```python
from build123d import *

# Parameters (mm, degrees)
SKETCH1_R           = 2
BOSS_EXTRUDE1_DEPTH = 2
SKETCH6_R           = 1.4
CUT_EXTRUDE1_DEPTH  = 10


with BuildPart() as part:
    # Sketch1 → Boss-Extrude1 (new body)
    with BuildSketch(Plane(origin=(0, 0, 0), x_dir=(1, 0, 0), z_dir=(0, 1, 0))):
        with BuildLine():
            ThreePointArc((9.383115236, 31.116027196), (-30.08527478, 12.293341344), (-15.092629238, -28.783025253))
            ThreePointArc((-15.092629238, -28.783025253), (-13.079214236, -32.008527478), (-9.383115236, -31.116027196))
            ThreePointArc((-9.383115236, -31.116027196), (30.08527478, -12.293341344), (15.092629238, 28.783025253))
            ThreePointArc((15.092629238, 28.783025253), (13.079214236, 32.008527478), (9.383115236, 31.116027196))
        make_face()
        with Locations((11.849880102, 29)):
            Circle(SKETCH1_R, mode=Mode.SUBTRACT)
        with Locations((-11.849880102, -29)):
            Circle(SKETCH1_R, mode=Mode.SUBTRACT)
    extrude(amount=BOSS_EXTRUDE1_DEPTH)

    # Sketch6 → Cut-Extrude1 (cut)
    with BuildSketch(Plane.XZ):
        with Locations((-21.83, -13.926611625)):
            Circle(SKETCH6_R)
        with Locations((22.12, 14.29)):
            Circle(SKETCH6_R)
    extrude(amount=-CUT_EXTRUDE1_DEPTH, mode=Mode.SUBTRACT)


solid = part.part
```
CAD build for the part. Positions are in the model's coordinates, mm. Coordinates: 2 decimals unless noted, no trailing zeros. Loops run counter-clockwise (first coordinate to the right, second up) from the corner with the lowest first, then second, coordinate; pieces in that order, holes last. Notation, with made-up numbers: (14.25, 77.25) - (26.25, 77.25) arc R22 ccw to (26.25, 99.25) - close; hole circle Ø7 at (-13, 66). An arc over 180 degrees is marked (long way). Return JSON: item names as keys, results as strings.
1. Band-saw the part on B-B (x = 12). Give the cut face in (y, z), and give its area (3 significant figures).
Result:
{"outline": "(0, -32.25) - (2, -32.25) - (2, -30.99) - (0, -30.99) - close; (0, -27.01) - (2, -27.01) - (2, 30.2) - (0, 30.2) - close", "area": "117 mm2"}
2. Band-saw the part on A-A (z = 14.29). Give the cut face in (x, y), and give its area (3 significant figures).
Result:
{"outline": "(-29.19, 0) - (20.72, 0) - (20.72, 2) - (-29.19, 2) - close; (23.52, 0) - (29.19, 0) - (29.19, 2) - (23.52, 2) - close", "area": "111 mm2"}
3. Mould opens along Z. For faces 1 (the cylindrical face through (29.825, 0.986, 12.912)), 2 (the cylindrical face through (-10.927, 0.986, 30.774)), 3 (the flat face through (0, 2, 0)) say: released by +Z, released by -Z, zero draft, split by the parting line, or undercut.
Result:
{"face 1": "split by the parting line", "face 2": "undercut", "face 3": "zero draft"}
4. Probe L1, parallel to X at y = 0.3, z = 4; L2, parallel to Z at x = 0.5, y = 0.95; L3, parallel to Z at x = -21.83, y = 1.1. List the from-to ranges inside material, lowest first. Write a range as from..to.
Result:
{"L1": "x = -32.25..32.25", "L2": "z = -32.5..32.5", "L3": "z = -24.08..-15.33, -12.53..24.08"}
5. Band-saw the part on C-C (y = 1.45). Give the cut face in (x, z), and give its area (3 significant figures).
Result:
{"outline": "(-15.09, 28.78) arc R32.5 ccw to (9.38, -31.12) arc R3.25 ccw to (15.09, -28.78) arc R32.5 ccw to (-9.38, 31.12) arc R3.25 ccw to start; hole circle Ø2.8 at (-21.83, -13.93); hole circle Ø4 at (-11.85, 29); hole circle Ø4 at (11.85, -29); hole circle Ø2.8 at (22.12, 14.29)", "area": "3,300 mm2"}
6. Band-saw the part on D-D (x = -27). Give the cut face in (y, z), and give its area (3 significant figures).
Result:
{"outline": "(0, -18.09) - (2, -18.09) - (2, 18.09) - (0, 18.09) - close", "area": "72.4 mm2"}
